Read the model definition and answer for the solid it produces. Units are mm, in the model's axes. Round coordinates to 2 decimals unless told otherwise and drop trailing zeros. Write each loop counter-clockwise with the first axis right and the second up, starting at its lowest first coordinate (ties: lowest second). Pieces come first, ordered by that corner, then holes.
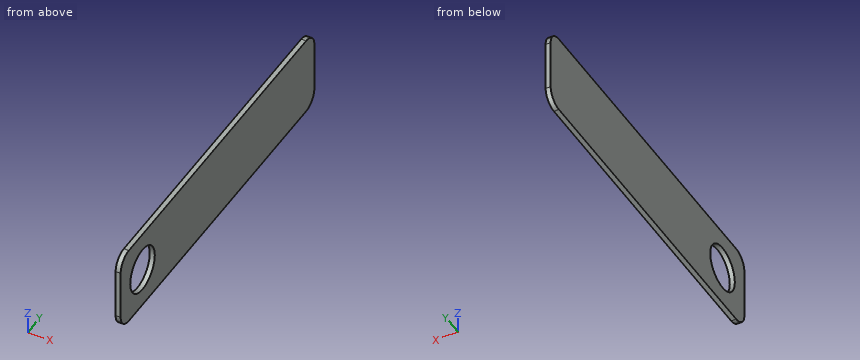
from build123d import *

# Parameters (mm, degrees)
SKETCH1_W           = 50.8
SKETCH1_H           = 225.425
SKETCH1_R           = 14.2875
BOSS_EXTRUDE1_DEPTH = 3.175
FILLET1_R           = 9.525


with BuildPart() as part:
    # Sketch1 → Boss-Extrude1 (new body)
    with BuildSketch(Plane(origin=(0, 0, 0), x_dir=(0, 0, -1), z_dir=(1, 0, 0))):
        Rectangle(SKETCH1_W, SKETCH1_H)
        with Locations((0, -87.3125)):
            Circle(SKETCH1_R, mode=Mode.SUBTRACT)
    extrude(amount=BOSS_EXTRUDE1_DEPTH)

    # Fillet1
    fillet1_edges = [part.edges().sort_by_distance(p)[0] for p in [
        (1.5875, 112.7125, 25.4),
        (1.5875, 112.7125, -25.4),
        (1.5875, -112.7125, -25.4),
        (1.5875, -112.7125, 25.4),
    ]]
    fillet(fillet1_edges, radius=FILLET1_R)


solid = part.part
Q1. Section C-C (y = -84.5) is taken. Determine the outline of the cut face in (x, z) (3 decimals), then the cut area to 3 significant figures.
Verdict:
outline: (0, -25.4) - (3.175, -25.4) - (3.175, -14.008) - (0, -14.008) - close; (0, 14.008) - (3.175, 14.008) - (3.175, 25.4) - (0, 25.4) - close
area: 72.3 mm2
Q2. Straight lines are drawn through the part: probe 1 along Y at (x, z) = (0.7, 0) (1 decimal); probe 2 along Z at (x, y) = (2.8, -75.5); probe 3 along Y at (x, z) = (2.35, -5). For each, find the intervals that lie inside material, in ascending order.
Verdict:
probe 1: y = -112.7 to -101.6, -73 to 112.7
probe 2: z = -25.4 to -8.04, 8.04 to 25.4
probe 3: y = -112.71 to -100.7, -73.93 to 112.71
Q3. Section A-A (z = 0) is taken. Determine the outline of the cut face in (x, y) (1 decimal).
Verdict:
outline: (0, -112.7) - (3.2, -112.7) - (3.2, -101.6) - (0, -101.6) - close; (0, -73) - (3.2, -73) - (3.2, 112.7) - (0, 112.7) - close
Q4. A flat-ended cylindrical pin translates along its axis: pin 1 Ø17 at (y, z) = (-87.31, 0) entering from +X. Find the tip coordinate at first contact, or state that the pin passes through.
Verdict:
pin 1: passes through
